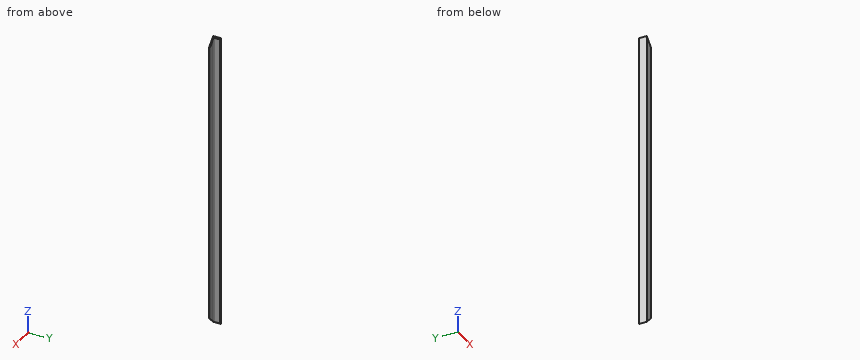
Autodesk Inventor part; units mm, degrees
ref_plane "Start Plane" through (0, 0, 0) normal (0, 0, 1) x (1, 0, 0)
ref_plane "End Plane" through (0, 0, 979.0722) normal (0, 0, 1) x (1, 0, 0)
ref_plane "Work Plane4" through (0, 12.7, 0) normal (0.7071, 0, -0.7071) x (-0.7071, 0, -0.7071)
ref_plane "Start Plane" through (0, 0, 0) normal (0, 0, 1) x (1, 0, 0)
ref_plane "End Plane" through (0, 0, 979.0722) normal (0, 0, 1) x (1, 0, 0)
sketch "Sketch" plane through (0, 0, 0) normal (0, 0, 1) x (1, 0, 0)
  line L0 (25.4, 0) -> (0, 0)
  line L1 (0, 0) -> (0, 25.4)
  line L2 (0, 25.4) -> (1.651, 25.4)
  line L3 (3.175, 23.876) -> (3.175, 6.477)
  line L4 (6.477, 3.175) -> (23.876, 3.175)
  line L5 (25.4, 1.651) -> (25.4, 0)
  line L6 (0, -11.0414) -> (0, 31.5385) construction
  line L7 (-11.0414, 0) -> (31.5385, 0) construction
  arc A0 (3.175, 6.477) -> (6.477, 3.175) centre (6.477, 6.477) ccw
  arc A1 (3.175, 23.876) -> (1.651, 25.4) centre (1.651, 23.876) ccw
  arc A2 (25.4, 1.651) -> (23.876, 3.175) centre (23.876, 1.651) ccw
  line L8 (0, 40.0545) -> (0, -19.5574) construction
  line L9 (-19.5574, 0) -> (40.0545, 0) construction
  point P0 (3.175, 25.4)
  point P1 (3.175, 3.175)
  point P2 (25.4, 3.175)
  dimension "d0" = 25.4
  dimension "d1" = 25.4
  dimension "d2" = 3.175
  dimension "d3" = 3.175
  dimension "d10" = 0
  dimension "d11" = 0
  dimension "d14" = 3.302
  dimension "d15" = 1.524
extrude "Body" add sketch "Sketch" along normal up to surface (979.0722 mm away) from surface at 0
sketch "Sketch3" plane through (0, 0, 0) normal (0, 0, 1) x (1, 0, 0)
  line L0 (0, 0) -> (10, 0)
ref_plane "Work Plane3" through (0, 0, 0) normal (0, -1, 0) x (1, 0, 0)
ref_plane "Work Plane4" through (0, 12.7, 0) normal (0.7071, 0, -0.7071) x (-0.7071, 0, -0.7071)
split "Split1" plane through (0, 12.7, 0) removes the side toward (0.7071, 0, -0.7071)
ref_plane "Work Plane5" through (0, 12.7, 979.0722) normal (0.7071, 0, 0.7071) x (0.7071, 0, -0.7071)
split "Split2" plane through (0, 12.7, 979.0722) removes the side toward (0.7071, 0, 0.7071)
sketch "Sketch4" plane through (0, 0, 0) normal (0, -1, 0) x (1, 0, 0)
  line L0 (-2, 0) -> (12, 0)
  line L1 (-2, 979.0722) -> (12, 979.0722)
  dimension "d17" = 979.0722
equation "\"d0\" = G_H"
equation "\"d1\" = G_H"
equation "\"d2\" = G_T"
equation "\"d3\" = G_T"
equation "\"d14\" = G_IR"
equation "\"d15\" = G_ER"
equation "\"d4\" = G_L"
equation "\"G_H\" = 25.4"
equation "\"G_T\" = 3.175"
equation "\"G_ER\" = 1.524"
equation "\"G_IR\" = 3.302"
equation "\"G_L\" = d17"
equation "\"ex\" = 0"
equation "\"G_OFFSET_START\" = 0"
equation "\"G_OFFSET_END\" = 0"
equation "\"d13\" = G_OFFSET_END + B_L"
equation "\"B_L\" = 979.07217"
properties part number "AISC - L 1 x 1 x 1/8 - 38.546" material "Steel, Mild"
Here's how the part is built. I have some questions about the finished solid (model axes, mm). Round coordinates to 2 decimals unless told otherwise and drop trailing zeros. Write each loop counter-clockwise with the first axis right and the second up, starting at its lowest first coordinate (ties: lowest second). Pieces come first, ordered by that corner, then holes.
1. I need wall thicknesses on L1, parallel to Y at x = 22.25, z = 381 (3 decimals); L2, parallel to X at y = 1.75, z = 530. Which ranges of each line are inside material? Lowest first, please.
2. Will these pins go through, and if not, where does the flat tip stop? pin 1 Ø5 at (y, z) = (19, 258) entering from +X (3 decimals); pin 2 Ø8.5 at (x, z) = (19.5, 723.5) entering from +Y (3 decimals); pin 3 Ø10 at (x, y) = (7.5, 19) entering from +Z.
3. Suppose I cut it at C-C (x = 15.25). List the corners of the cut face in (y, z) for me (3 decimals), and give its area (3 significant figures).
4. Suppose I cut it at A-A (z = 306.5). List the corners of the cut face in (x, y) for me (3 decimals).
5. Suppose I cut it at B-B (y = 11.25). List the corners of the cut face in (x, z) for me (3 decimals), and give its area (3 significant figures).
Answer sheet:
1. L1: y = 0 to 3.175
1. L2: x = 0 to 25.4
2. pin 1: stops at x = 3.175
2. pin 2: stops at y = 3.175
2. pin 3: stops at z = 976.57
3. outline: (0, 15.25) - (3.175, 15.25) - (3.175, 963.822) - (0, 963.822) - close
3. area: 3,010 mm2
4. outline: (0, 0) - (25.4, 0) - (25.4, 1.651) arc R1.524 ccw to (23.876, 3.175) - (6.477, 3.175) arc R3.302 cw to (3.175, 6.477) - (3.175, 23.876) arc R1.524 ccw to (1.651, 25.4) - (0, 25.4) - close
5. outline: (0, 0) - (3.175, 3.175) - (3.175, 975.897) - (0, 979.072) - close
5. area: 3,100 mm2
